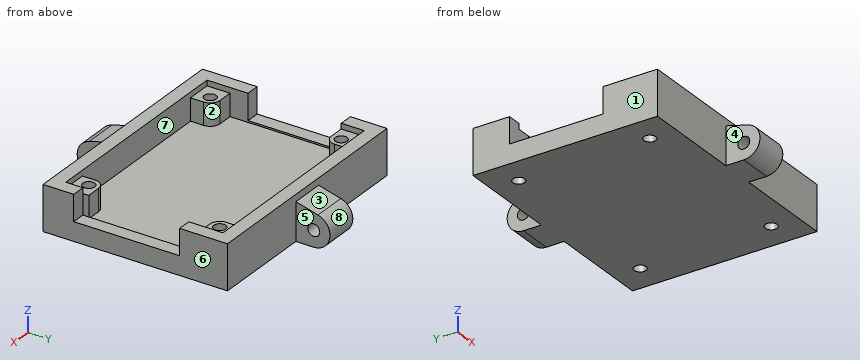
from build123d import *

# Parameters (mm, degrees)
SKETCH1_W           = 62
SKETCH1_H           = 46
SKETCH1_R           = 1.75
BOSS_EXTRUDE1_DEPTH = 5
SKETCH1_3_W         = 70
SKETCH1_3_H         = 54
SKETCH1_3_W_2       = 62
SKETCH1_3_H_2       = 46
BOSS_EXTRUDE2_DEPTH = 13.1
SKETCH2_W           = 12.7
SKETCH2_H           = 4
CUT_EXTRUDE1_DEPTH  = 4
SKETCH3_R           = 1.75
BOSS_EXTRUDE3_DEPTH = 6.5
SKETCH4_W           = 4
SKETCH4_H           = 27.275016295
SKETCH4_H_2         = 31
CUT_EXTRUDE2_DEPTH  = 7.6
SKETCH5_R           = 1.75
BOSS_EXTRUDE4_DEPTH = 5


with BuildPart() as part:
    # Sketch1 → Boss-Extrude1 (new body)
    with BuildSketch(Plane.XY):
        Rectangle(SKETCH1_W, SKETCH1_H)
        with Locations((26.638347595, -19.175016295)):
            Circle(SKETCH1_R, mode=Mode.SUBTRACT)
        with Locations((26.638347595, 19.175016295)):
            Circle(SKETCH1_R, mode=Mode.SUBTRACT)
        with Locations((-26.638347595, 19.175016295)):
            Circle(SKETCH1_R, mode=Mode.SUBTRACT)
        with Locations((-26.638347595, -19.175016295)):
            Circle(SKETCH1_R, mode=Mode.SUBTRACT)
    extrude(amount=BOSS_EXTRUDE1_DEPTH)

    # Sketch1<3> → Boss-Extrude2 (add)
    with BuildSketch(Plane.XY):
        Rectangle(SKETCH1_3_W, SKETCH1_3_H)
        Rectangle(SKETCH1_3_W_2, SKETCH1_3_H_2, mode=Mode.SUBTRACT)
    extrude(amount=BOSS_EXTRUDE2_DEPTH)

    # Sketch2 → Cut-Extrude1 (cut)
    with BuildSketch(Plane.XY.offset(5)):
        with Locations((-3.48328221, 21)):
            Rectangle(SKETCH2_W, SKETCH2_H)
    extrude(amount=-CUT_EXTRUDE1_DEPTH, mode=Mode.SUBTRACT)

    # Sketch3 → Boss-Extrude3 (add)
    # profile 1 of 4: a face of its own
    with BuildSketch(Plane.XY.offset(5)):
        with BuildLine():
            Line((-23.738347595, 19.175016295), (-23.738347595, 23))
            Line((-23.738347595, 23), (-31, 23))
            Line((-31, 23), (-31, 16.275016295))
            Line((-31, 16.275016295), (-26.638347595, 16.275016295))
            ThreePointArc((-26.638347595, 16.275016295), (-24.58773793, 17.12440663), (-23.738347595, 19.175016295))
        make_face()
        with Locations((-26.638347595, 19.175016295)):
            Circle(SKETCH3_R, mode=Mode.SUBTRACT)
    # profile 2 of 4: a face of its own
    with BuildSketch(Plane.XY.offset(5)):
        with BuildLine():
            Line((-31, -16.275016295), (-26.638347595, -16.275016295))
            ThreePointArc((-26.638347595, -16.275016295), (-24.58773793, -17.12440663), (-23.738347595, -19.175016295))
            Line((-23.738347595, -19.175016295), (-23.738347595, -23))
            Line((-23.738347595, -23), (-31, -23))
            Line((-31, -23), (-31, -16.275016295))
        make_face()
        with Locations((-26.638347595, -19.175016295)):
            Circle(SKETCH3_R, mode=Mode.SUBTRACT)
    # profile 3 of 4: a face of its own
    with BuildSketch(Plane.XY.offset(5)):
        with BuildLine():
            Line((31, -23), (31, -16.275016295))
            Line((31, -16.275016295), (26.638347595, -16.275016295))
            ThreePointArc((26.638347595, -16.275016295), (24.58773793, -17.12440663), (23.738347595, -19.175016295))
            Line((23.738347595, -19.175016295), (23.738347595, -23))
            Line((23.738347595, -23), (31, -23))
        make_face()
        with Locations((26.638347595, -19.175016295)):
            Circle(SKETCH3_R, mode=Mode.SUBTRACT)
    # profile 4 of 4: a face of its own
    with BuildSketch(Plane.XY.offset(5)):
        with BuildLine():
            Line((31, 16.275016295), (26.638347595, 16.275016295))
            ThreePointArc((26.638347595, 16.275016295), (24.58773793, 17.12440663), (23.738347595, 19.175016295))
            Line((23.738347595, 19.175016295), (23.738347595, 23))
            Line((23.738347595, 23), (31, 23))
            Line((31, 23), (31, 16.275016295))
        make_face()
        with Locations((26.638347595, 19.175016295)):
            Circle(SKETCH3_R, mode=Mode.SUBTRACT)
    extrude(amount=BOSS_EXTRUDE3_DEPTH)

    # Sketch4 → Cut-Extrude2 (cut)
    with BuildSketch(Plane.XY.offset(13.1)):
        with Locations((-33, 2.637508148)):
            Rectangle(SKETCH4_W, SKETCH4_H)
        with Locations((33, -2.5)):
            Rectangle(SKETCH4_W, SKETCH4_H_2)
    extrude(amount=-CUT_EXTRUDE2_DEPTH, mode=Mode.SUBTRACT)

    # Sketch5 → Boss-Extrude4 (add, symmetric)
    # profile 1 of 2: a face of its own
    with BuildSketch(Plane(origin=(0, 0, 0), x_dir=(0, 0, -1), z_dir=(1, 0, 0))):
        with BuildLine():
            Line((-11.074295117, 27), (-9.338147675, 33.479390464))
            ThreePointArc((-9.338147675, 33.479390464), (-4.130000587, 36.959363092), (0, 32.25))
            Line((0, 32.25), (0, 27))
            Line((0, 27), (-11.074295117, 27))
        make_face()
        with Locations((-4.75, 32.25)):
            Circle(SKETCH5_R, mode=Mode.SUBTRACT)
    # profile 2 of 2: a face of its own
    with BuildSketch(Plane(origin=(0, 0, 0), x_dir=(0, 0, -1), z_dir=(1, 0, 0))):
        with BuildLine():
            Line((0, -32.25), (0, -27))
            Line((0, -27), (-11.074295117, -27))
            Line((-11.074295117, -27), (-9.338147675, -33.479390464))
            ThreePointArc((-9.338147675, -33.479390464), (-4.130000587, -36.959363092), (0, -32.25))
        make_face()
        with Locations(Location((-4.75, -32.25, 0), (0, 0, 180))):
            Circle(SKETCH5_R, mode=Mode.SUBTRACT)
    extrude(amount=BOSS_EXTRUDE4_DEPTH, both=True)


solid = part.part
Geometry check sheet. Reference: the model listing, model coordinates, mm. Face numbers are marked on the shaded views. A direction names the side the tool comes from. Coordinates: 2 decimals unless noted, no trailing zeros. Write each loop counter-clockwise with the first axis right and the second up, starting at its lowest first coordinate (ties: lowest second). Pieces come first, ordered by that corner, then holes. Notation, with made-up numbers: (-25.75, 21) -> (-14.75, 21) arc R15 cw to (-14.75, 27) -> close; hole circle Ø4 at (-35, 77). An arc over 180 degrees is marked (long way). One line per question, with ' | ' between items.
1. Cross-section at D-D on z = 8. State how many separate pieces and enclosed holes the cut face has, and give its area (3 significant figures).
Answers:
separate pieces: 2 | enclosed holes: 4 | area: 1,020 mm²
2. Depth check by flat-ended pin: pin 1 Ø4 at (x, z) = (2.5, 9.5) entering from -Y; pin 2 Ø5 at (x, y) = (0.5, -17) entering from +Z; pin 3 Ø3.5 at (x, z) = (29.5, 8) entering from -Y; pin 4 Ø2 at (x, y) = (26.64, 19.18) entering from -Z. Enter the tip coordinate at first touch or a pass-through.
Answers:
pin 1: stops at y = -36.12 | pin 2: stops at z = 5 | pin 3: stops at y = -27 | pin 4: passes through
3. Thickness scan on probe 1 along X at (y, z) = (-19, 1.75); probe 2 along X at (y, z) = (-21.5, 12.5); probe 3 along Y at (x, z) = (-20.5, 6). Record the ranges inside material, lowest first. Write a range as from..to.
Answers:
probe 1: x = -35..-28.38, -24.9..24.9, 28.38..35 | probe 2: x = -35..-31, 31..35 | probe 3: y = -27..-23, 23..27
4. Set-up check for the marked faces 4, 5, 6, 7 and 8: record each of +Z, -Z, +X, -X, +Y, -Y from which the full face is reachable in a straight line by a thin tool's end or side.
Answers:
face 4: +Z, -Z, -X, -Y | face 5: +Z, -Z, +X, +Y | face 6: +Z, -Z, +X, +Y, -Y | face 7: +Z | face 8: +X, -X, +Y
5. Cross-section at A-A on z = 4. Record the cut outline in (x, y), and give its area (3 significant figures).
Answers:
outline: (-35, -27) -> (-5, -27) -> (-5, -30.67) -> (5, -30.67) -> (5, -27) -> (35, -27) -> (35, 27) -> (5, 27) -> (5, 30.67) -> (-5, 30.67) -> (-5, 27) -> (-35, 27) -> close; (-5, -36.94) -> (5, -36.94) -> (5, -33.83) -> (-5, -33.83) -> close; (-5, 33.83) -> (5, 33.83) -> (5, 36.94) -> (-5, 36.94) -> close; hole circle Ø3.5 at (-26.64, -19.18); hole circle Ø3.5 at (-26.64, 19.18); hole (-9.83, 19) -> (2.87, 19) -> (2.87, 23) -> (-9.83, 23) -> close; hole circle Ø3.5 at (26.64, -19.18); hole circle Ø3.5 at (26.64, 19.18) | area: 3,830 mm²
6. Draft check along X on the marked faces 1, 2 and 3. Enter one of: +X half, -X half, draft (parallel to the pull), parting line (faces both ways), or undercut.
Answers:
face 1: -X half | face 2: undercut | face 3: draft
7. Cross-section at B-B on x = -19. Record the cut outline in (y, z).
Answers:
outline: (-27, 0) -> (27, 0) -> (27, 13.1) -> (23, 13.1) -> (23, 5) -> (-23, 5) -> (-23, 13.1) -> (-27, 13.1) -> close
8. Cross-section at C-C on y = -10. Record the cut outline in (x, z).
Answers:
outline: (-35, 0) -> (35, 0) -> (35, 5.5) -> (31, 5.5) -> (31, 5) -> (-31, 5) -> (-31, 5.5) -> (-35, 5.5) -> close
